Geometry check sheet. Reference: the model listing, model coordinates, mm. Face numbers are marked on the shaded views. A direction names the side the tool comes from. Give positions to 0.01 mm unless a question says otherwise; leave off trailing zeros. Write each loop counter-clockwise with the first axis right and the second up, starting at its lowest first coordinate (ties: lowest second). Pieces come first, ordered by that corner, then holes. Notation, with made-up numbers: (-0.75, 11) - (7.25, 11) arc R26 ccw to (7.25, 39) - close; hole circle Ø6 at (3.25, 11). An arc over 180 degrees is marked (long way). One line per question, with ' | ' between items. Start each with the question number.
Q1. Section check D-D on y = 52.5. Record the boundary of the cut face in (x, z).
Q2. Section check B-B on z = 130. Record the boundary of the cut face in (x, y).
Q3. Section check A-A on y = 12. Record the boundary of the cut face in (x, z).
Q4. Set-up check for the marked faces 1, 2, 3 and 4: record each of +Z, -Z, +X, -X, +Y, -Y from which the full face is reachable in a straight line by a thin tool's end or side.
Q5. Gauge pin test, flat ends, axial feed: P1, Ø1, axis at x = -106, z = 30.5, coming from the -Y side; P2, Ø8, axis at y = 5.5, z = 73.5, coming from the -X side; P3, Ø5, axis at x = 26, y = 86.5, coming from the -Z side. Record the tip position at first contact, or that the pin passes through.
Q6. Section check C-C on x = -19. Record the boundary of the cut face in (y, z).
Q7. Thickness scan on L1, parallel to Z at x = 83.5, y = 36.5; L2, parallel to X at y = 4, z = 122.5; L3, parallel to Y at x = 3.5, z = -41. Record the ranges inside material, lowest first. Write a range as [from, to].
Autodesk Inventor part; units mm, degrees
ref_plane "YZ Plane" through (0, 0, 0) normal (1, 0, 0) x (0, 1, 0)
ref_plane "XZ Plane" through (0, 0, 0) normal (0, 1, 0) x (-1, 0, 0)
ref_plane "XY Plane" through (0, 0, 0) normal (0, 0, 1) x (1, 0, 0)
sketch "Boceto1" plane through (0, 0, 0) normal (0, 1, 0) x (-1, 0, 0)
  line L0 (-121, -177.5) -> (121, -177.5)
  line L1 (121, -177.5) -> (121, 177.5)
  line L2 (121, 177.5) -> (-121, 177.5)
  line L3 (-121, 177.5) -> (-121, -177.5)
  line L4 (-121, -177.5) -> (121, 177.5) construction
  line L5 (121, -177.5) -> (-121, 177.5) construction
  point P0 (0, 0)
  dimension "d0" = 242
  dimension "d1" = 355
extrude "Extrusión1" add sketch "Boceto1" along normal blind 105
sketch "Boceto2" plane through (0, 105, 0) normal (0, 1, 0) x (1, 0, 0)
  line L0 (-121, 177.5) -> (-121, -177.5)
  line L1 (-121, -177.5) -> (121, -177.5)
  line L2 (121, -177.5) -> (121, 177.5)
  line L3 (121, 177.5) -> (-121, 177.5)
  line L4 (107, -163.5) -> (-107, -163.5)
  line L5 (-107, -163.5) -> (-107, 163.5)
  line L6 (-107, 163.5) -> (107, 163.5)
  line L7 (107, 163.5) -> (107, -163.5)
  point P0 (0, 0)
  dimension "d4" = 14
extrude "Extrusión2" cut sketch "Boceto2" against normal blind 86 contours L4 L5 L6 L7
sketch "Boceto3" plane through (0, 0, 0) normal (0, -1, 0) x (1, 0, 0)
  line L0 (-121, -177.5) -> (-121, 177.5)
  line L1 (121, -177.5) -> (-121, -177.5)
  line L2 (121, 177.5) -> (121, -177.5)
  line L3 (-121, 177.5) -> (121, 177.5)
  line L4 (107, 163.5) -> (107, -163.5)
  line L5 (107, -163.5) -> (-107, -163.5)
  line L6 (-107, -163.5) -> (-107, 163.5)
  line L7 (-107, 163.5) -> (107, 163.5)
  point P0 (0, 0)
  dimension "d7" = 14
extrude "Extrusión3" cut sketch "Boceto3" against normal blind 16 contours L4 L5 L6 L7
sketch "Boceto4" plane through (-121, 0, -177.5) normal (-1, 0, 0) x (0, 0, 1)
  line L0 (0, 0) -> (355, 0)
  line L1 (355, 0) -> (355, 105)
  line L2 (0, 105) -> (355, 105)
  line L3 (0, 0) -> (0, 105)
  line L4 (355, 105) -> (355, 117)
  line L5 (355, 105) -> (367, 105) construction
  line L6 (355, 117) -> (367, 117)
  line L7 (0, 0) -> (-12, 0)
  line L8 (-12, 0) -> (-12, -12)
  line L9 (-12, -12) -> (367, -12)
  line L10 (367, -12) -> (367, 117)
  line L11 (367, 117) -> (-12, 117)
  line L12 (-12, 117) -> (-12, -12)
  point P0 (177.5, 0)
  point P1 (-12, 0)
  dimension "d10" = 12
  dimension "d11" = 90
  dimension "d12" = 12
  dimension "d13" = 90
  dimension "d14" = 12
  dimension "d15" = 12
  dimension "d16" = 90
extrude "Extrusión4" add sketch "Boceto4" along normal blind 15
sketch "Boceto5" plane through (-136, 0, -177.5) normal (-1, 0, 0) x (0, 0, 1)
  line L0 (-12, 117) -> (-12, -12)
  line L1 (-12, -12) -> (367, -12)
  line L2 (367, -12) -> (367, 117)
  line L3 (367, 117) -> (-12, 117)
  line L4 (-12, -12) -> (367, 117)
  circle A0 centre (177.5, 52.5) radius 10
  point P0 (177.5, 0)
  dimension "d19" = 20
extrude "Extrusión5" add sketch "Boceto5" along normal blind 30 contours A0 L4 | L4 A0
properties part number "Cajon"
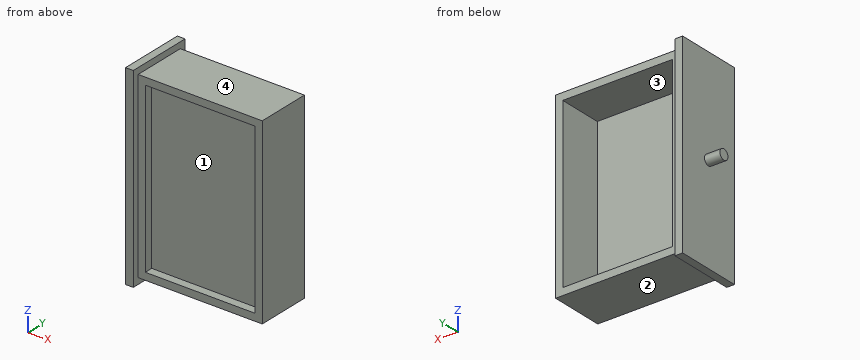
Working result:
1) outline: (-166, -10) - (-136, -10) - (-136, -189.5) - (-121, -189.5) - (-121, -177.5) - (121, -177.5) - (121, 177.5) - (-121, 177.5) - (-121, 189.5) - (-136, 189.5) - (-136, 10) - (-166, 10) - close; hole (-107, -163.5) - (107, -163.5) - (107, 163.5) - (-107, 163.5) - close
2) outline: (-136, -12) - (-121, -12) - (-121, 0) - (-107, 0) - (-107, 16) - (107, 16) - (107, 0) - (121, 0) - (121, 105) - (107, 105) - (107, 19) - (-107, 19) - (-107, 105) - (-121, 105) - (-121, 117) - (-136, 117) - close
3) outline: (-136, -189.5) - (-121, -189.5) - (-121, -177.5) - (121, -177.5) - (121, 177.5) - (-121, 177.5) - (-121, 189.5) - (-136, 189.5) - close; hole (-107, -163.5) - (107, -163.5) - (107, 163.5) - (-107, 163.5) - close
4) face 1: -Y | face 2: -Z, +X, +Y, -Y | face 3: +Y | face 4: +Z, +X, +Y, -Y
5) P1: stops at y = 16 | P2: stops at x = -136 | P3: stops at z = -177.5
6) outline: (0, -177.5) - (105, -177.5) - (105, -163.5) - (19, -163.5) - (19, 163.5) - (105, 163.5) - (105, 177.5) - (0, 177.5) - (0, 163.5) - (16, 163.5) - (16, -163.5) - (0, -163.5) - close
7) L1: z = [-177.5, -163.5], [163.5, 177.5] | L2: x = [-136, -107], [107, 121] | L3: y = [16, 19]
